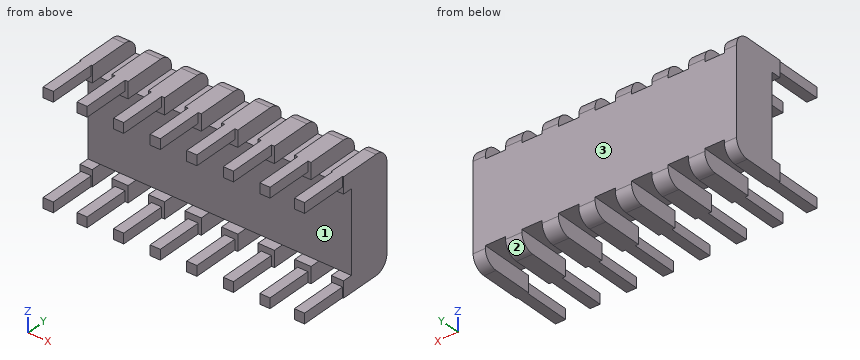
from build123d import *

# Parameters (mm, degrees)
SKETCH1_W           = 19.45
SKETCH1_H           = 6
BOSS_EXTRUDE1_DEPTH = 3.27
SKETCH2_W           = 0.9
SKETCH2_H           = 1.2
SKETCH2_W_2         = 1.2
BOSS_EXTRUDE2_DEPTH = 4
FILLET1_R           = 1
SKETCH3_W           = 0.75
SKETCH3_H           = 0.75
BOSS_EXTRUDE3_DEPTH = 3.5


with BuildPart() as part:
    # Sketch1 → Boss-Extrude1 (new body)
    with BuildSketch(Plane(origin=(0, 0, 0), x_dir=(1, 0, 0), z_dir=(0, 1, 0))):
        with Locations((9.725, 3)):
            Rectangle(SKETCH1_W, SKETCH1_H)
    extrude(amount=BOSS_EXTRUDE1_DEPTH)

    # Sketch2 → Boss-Extrude2 (add)
    with BuildSketch(Plane(origin=(0, 3.27, 0), x_dir=(1, 0, 0), z_dir=(0, 1, 0))):
        with Locations((19, -0.6)):
            Rectangle(SKETCH2_W, SKETCH2_H)
        with Locations((16.45, -0.6)):
            Rectangle(SKETCH2_W_2, SKETCH2_H)
        with Locations((13.75, -0.6)):
            Rectangle(SKETCH2_W_2, SKETCH2_H)
        with Locations((11.05, -0.6)):
            Rectangle(SKETCH2_W_2, SKETCH2_H)
        with Locations((8.35, -0.6)):
            Rectangle(SKETCH2_W_2, SKETCH2_H)
        with Locations((5.65, -0.6)):
            Rectangle(SKETCH2_W_2, SKETCH2_H)
        with Locations((2.95, -0.6)):
            Rectangle(SKETCH2_W_2, SKETCH2_H)
        with Locations((0.45, -0.6)):
            Rectangle(SKETCH2_W, SKETCH2_H)
        with Locations((0.45, 6.6)):
            Rectangle(SKETCH2_W, SKETCH2_H)
        with Locations((2.95, 6.6)):
            Rectangle(SKETCH2_W_2, SKETCH2_H)
        with Locations((5.65, 6.6)):
            Rectangle(SKETCH2_W_2, SKETCH2_H)
        with Locations((8.35, 6.6)):
            Rectangle(SKETCH2_W_2, SKETCH2_H)
        with Locations((11.05, 6.6)):
            Rectangle(SKETCH2_W_2, SKETCH2_H)
        with Locations((13.75, 6.6)):
            Rectangle(SKETCH2_W_2, SKETCH2_H)
        with Locations((16.45, 6.6)):
            Rectangle(SKETCH2_W_2, SKETCH2_H)
        with Locations((19, 6.6)):
            Rectangle(SKETCH2_W, SKETCH2_H)
    extrude(amount=-BOSS_EXTRUDE2_DEPTH)

    # Fillet1
    fillet1_edges = [part.edges().sort_by_distance(p)[0] for p in [
        (0.45, 3.27, 1.2),
        (0.45, 3.27, -7.2),
        (2.95, 3.27, -7.2),
        (5.65, 3.27, -7.2),
        (8.35, 3.27, -7.2),
        (19, 3.27, 1.2),
        (11.05, 3.27, -7.2),
        (13.75, 3.27, -7.2),
        (16.45, 3.27, -7.2),
        (19, 3.27, -7.2),
        (16.45, 3.27, 1.2),
        (13.75, 3.27, 1.2),
        (11.05, 3.27, 1.2),
        (8.35, 3.27, 1.2),
        (5.65, 3.27, 1.2),
        (2.95, 3.27, 1.2),
    ]]
    fillet(fillet1_edges, radius=FILLET1_R)

    # Sketch3 → Boss-Extrude3 (add)
    with BuildSketch(Plane.XZ.offset(0.73)):
        with Locations((19, 0.825)):
            Rectangle(SKETCH3_W, SKETCH3_H)
        with Locations((16.45, 0.825)):
            Rectangle(SKETCH3_W, SKETCH3_H)
        with Locations((13.75, 0.825)):
            Rectangle(SKETCH3_W, SKETCH3_H)
        with Locations((11.05, 0.825)):
            Rectangle(SKETCH3_W, SKETCH3_H)
        with Locations((8.35, 0.825)):
            Rectangle(SKETCH3_W, SKETCH3_H)
        with Locations((5.65, 0.825)):
            Rectangle(SKETCH3_W, SKETCH3_H)
        with Locations((2.95, 0.825)):
            Rectangle(SKETCH3_W, SKETCH3_H)
        with Locations((0.45, 0.825)):
            Rectangle(SKETCH3_W, SKETCH3_H)
        with Locations((0.45, -6.825)):
            Rectangle(SKETCH3_W, SKETCH3_H)
        with Locations((2.95, -6.825)):
            Rectangle(SKETCH3_W, SKETCH3_H)
        with Locations((5.65, -6.825)):
            Rectangle(SKETCH3_W, SKETCH3_H)
        with Locations((11.05, -6.825)):
            Rectangle(SKETCH3_W, SKETCH3_H)
        with Locations((8.35, -6.825)):
            Rectangle(SKETCH3_W, SKETCH3_H)
        with Locations((13.75, -6.825)):
            Rectangle(SKETCH3_W, SKETCH3_H)
        with Locations((16.45, -6.825)):
            Rectangle(SKETCH3_W, SKETCH3_H)
        with Locations((19, -6.825)):
            Rectangle(SKETCH3_W, SKETCH3_H)
    extrude(amount=BOSS_EXTRUDE3_DEPTH)


solid = part.part
Geometry: final body of the model. Coordinates: model frame, mm. Face numbers are marked on the shaded views. Give positions to 0.01 mm unless a question says otherwise; leave off trailing zeros. Write each loop counter-clockwise with the first axis right and the second up, starting at its lowest first coordinate (ties: lowest second). Pieces come first, ordered by that corner, then holes. Notation, with made-up numbers: (-4.5, 41) - (31.5, 41) arc R24 ccw to (31.5, 62) - close; hole circle Ø2 at (47, 77). An arc over 180 degrees is marked (long way). Return JSON: item names as keys, results as strings. Group by question number.
1) Section B-B on y = -2.75. State how many separate pieces and enclosed holes the cut face has, plus the area to 3 significant figures.
2) Mould query, pull axis Z, two halves, no side actions, for the marked faces 1, 2 and 3. Classes: released by +Z, released by -Z, zero draft, split by the parting line, or undercut.
3) Section C-C on z = -1.75. Return the cut outline in (x, y).
4) Section A-A on x = 16.5. Return the cut outline in (y, z), plus the area to 3 significant figures.
5) Line query: line 1 (Z direction, x = 3.25, y = -3.5); line 2 (Y direction, x = 16.25, z = -3); line 3 (Z direction, x = 5, y = 1.75). Output: solid intervals per line, ascending.
6) First-contact query: P1, Ø3, axis at x = 14.5, z = -5.5, coming from the -Y side; P2, Ø0.8, axis at y = -1.5, z = 0.5, coming from the -X side (3 decimals); P3, Ø0.8, axis at y = -2.5, z = -7, coming from the +X side (3 decimals); P4, Ø0.8, axis at x = 18, y = 2.5, coming from the +Z side. Flat tips, straight axial feed; report the tip coordinate or a pass-through.
Filled in:
{
 "1": {"separate pieces": "16", "enclosed holes": "0", "area": "9.00 mm^2"},
 "2": {"face 1": "undercut", "face 2": "released by -Z", "face 3": "zero draft"},
 "3": {"outline": "(0, 0) - (19.45, 0) - (19.45, 3.27) - (0, 3.27) - close"},
 "4": {"outline": "(-4.23, -7.2) - (2.27, -7.2) arc R1 ccw to (3.27, -6.2) - (3.27, 0.2) arc R1 ccw to (2.27, 1.2) - (-4.23, 1.2) - (-4.23, 0.45) - (-0.73, 0.45) - (-0.73, 0) - (0, 0) - (0, -6) - (-0.73, -6) - (-0.73, -6.45) - (-4.23, -6.45) - close", "area": "34.0 mm^2"},
 "5": {"line 1": "z = -7.2 to -6.45, 0.45 to 1.2", "line 2": "y = 0 to 3.27", "line 3": "z = -6 to 0"},
 "6": {"P1": "stops at y = -4.23", "P2": "stops at x = 0.075", "P3": "stops at x = 19.375", "P4": "stops at z = 0"}
}
